from build123d import *

# Parameters (mm, degrees)
BOSS_EXTRUDE1_DEPTH                 = 100
BOSS_EXTRUDE1_DEPTH_BACK            = 100
SKETCH3_R                           = 4
CHAMFER1_SIZE                       = 0.16
M6X1_0_TAPPED_HOLE1_D               = 5
M6X1_0_TAPPED_HOLE1_DEPTH           = 25
M6X1_0_TAPPED_HOLE1_TIP             = 1.502151548
M6X1_0_TAPPED_HOLE1_ON_FACE_2_D     = 5
M6X1_0_TAPPED_HOLE1_ON_FACE_2_DEPTH = 25
M6X1_0_TAPPED_HOLE1_ON_FACE_2_TIP   = 1.502151548


with BuildPart() as part:
    # Sketch3 → Boss-Extrude1 (new, two sides: drawn at the far end of the back side and taken through both)
    with BuildSketch(Plane.XY.offset(-BOSS_EXTRUDE1_DEPTH_BACK)):
        Circle(SKETCH3_R)
    extrude(amount=BOSS_EXTRUDE1_DEPTH + BOSS_EXTRUDE1_DEPTH_BACK)

    # Chamfer1
    chamfer1_edges = [part.edges().sort_by_distance(p)[0] for p in [
        (-4, 0, -100),
        (-4, 0, 100),
    ]]
    chamfer(chamfer1_edges, length=CHAMFER1_SIZE)

    # M6x1.0 Tapped Hole1
    with Locations(Plane.XY.offset(100)):
        with Locations((0, 0)):
            Hole(M6X1_0_TAPPED_HOLE1_D / 2, depth=M6X1_0_TAPPED_HOLE1_DEPTH)
            with Locations((0, 0, -(M6X1_0_TAPPED_HOLE1_DEPTH + M6X1_0_TAPPED_HOLE1_TIP / 2))):  # 118° drill point
                Cone(0, M6X1_0_TAPPED_HOLE1_D / 2, M6X1_0_TAPPED_HOLE1_TIP, mode=Mode.SUBTRACT)

    # M6x1.0 Tapped Hole1 on face 2
    with Locations(Plane(origin=(0, 0, -100), x_dir=(-1, 0, 0), z_dir=(0, 0, -1))):
        with Locations((0, 0)):
            Hole(M6X1_0_TAPPED_HOLE1_ON_FACE_2_D / 2, depth=M6X1_0_TAPPED_HOLE1_ON_FACE_2_DEPTH)
            with Locations((0, 0, -(M6X1_0_TAPPED_HOLE1_ON_FACE_2_DEPTH + M6X1_0_TAPPED_HOLE1_ON_FACE_2_TIP / 2))):  # 118° drill point
                Cone(0, M6X1_0_TAPPED_HOLE1_ON_FACE_2_D / 2, M6X1_0_TAPPED_HOLE1_ON_FACE_2_TIP, mode=Mode.SUBTRACT)


solid = part.part
Verification items for the finished model (mm, model axes). A direction names the side the tool comes from. Give positions to 0.01 mm unless a question says otherwise; leave off trailing zeros. Loops run counter-clockwise (first coordinate to the right, second up) from the corner with the lowest first, then second, coordinate; pieces in that order, holes last. Notation, with made-up numbers: (56.25, -18) - (101.25, -18) arc R36 cw to (101.25, 17) - close; hole circle Ø5 at (30.25, 85.25). An arc over 180 degrees is marked (long way). Write item = value, one per line. Start each with the question number.
Q1. Tool access check on faces 4 (the face through (0.54, -2.44, 87.32)), 5 (the face through (0.094, -0.424, -73.759)). Record the directions out of +Z, -Z, +X, -X, +Y, -Y that give a thin tool (end or side, any length) a straight path to the whole face; none if there is none.
Q2. Thickness scan on line 1 (Y direction, x = 0, z = 85.75); line 2 (X direction, y = -0.5, z = -56.5). Record the ranges inside material, lowest first.
Q3. Mould release check, pull along X, two halves, no side actions. Record for faces 1 (the face through (0, -3, -100)), 2 (the face through (-0.867, -3.905, -1.398)), 3 (the face through (-0.54, -2.44, -87.32)): released by +X, released by -X, zero draft, split by the parting line, or undercut.
Q4. Depth check by flat-ended pin: P1, Ø4.5, axis at x = 0, y = 0, coming from the +Z side. Enter the tip coordinate at first touch or a pass-through.
Q5. Cross-section at A-A, the plane z = 61. Enter the section's corners in (x, y).
Answer key:
q1.face_4 = +Z
q1.face_5 = -Z
q2.line_1 = -4 to -2.5, 2.5 to 4
q2.line_2 = -3.97 to 3.97
q3.face_1 = zero draft
q3.face_2 = split by the parting line
q3.face_3 = undercut
q4.P1 = 74.85
q5.outline = circle Ø8 at (0, 0)
